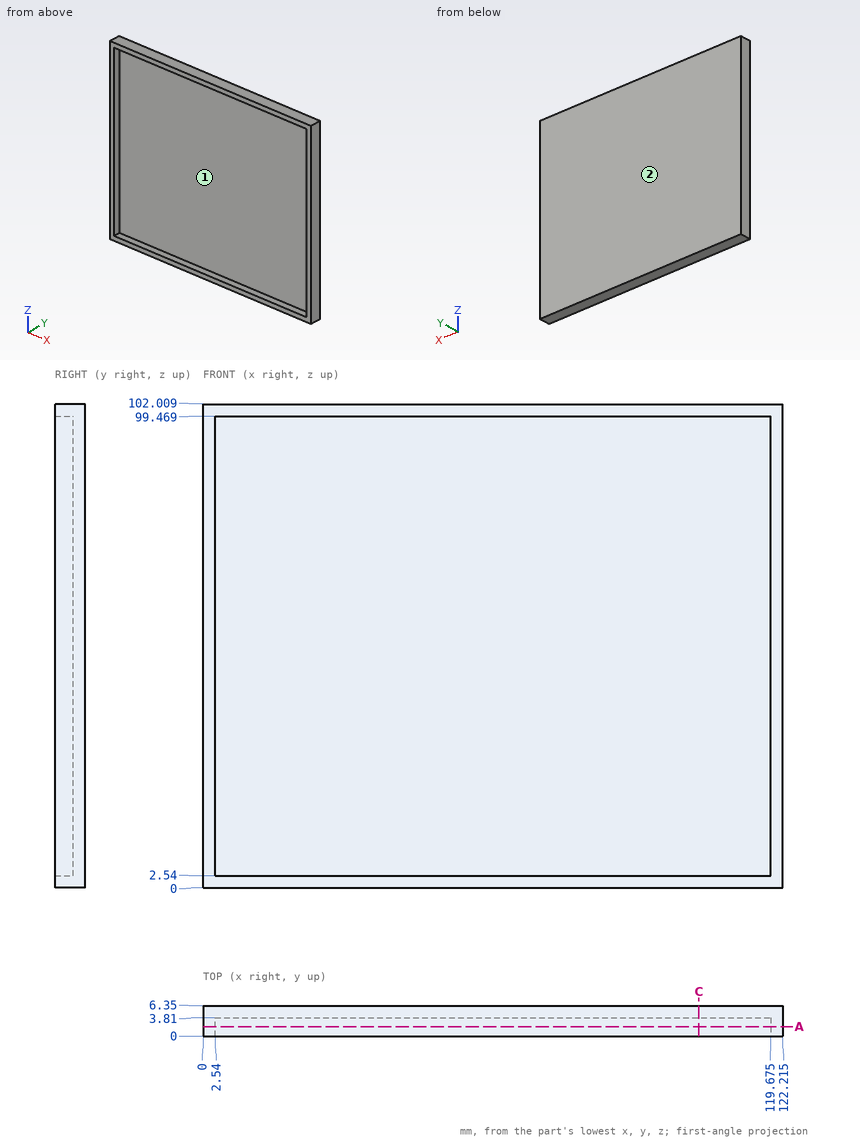
Can you work these out from the drawing? Everything is in mm from the part's minimum corner. Coordinates: 2 decimals unless noted, no trailing zeros. Write each loop counter-clockwise with the first axis right and the second up, starting at its lowest first coordinate (ties: lowest second). Pieces come first, ordered by that corner, then holes. Notation, with made-up numbers: (31, 52) -> (88, 52) arc R34 cw to (88, 86) -> close; hole circle Ø3 at (80.5, 22). An arc over 180 degrees is marked (long way). Write each question's results on one line, items separated by ' | '. Start each with the question number.
Item 1: If we section it at C-C, the plane x = 104.5: Write out the boundary of the cut face in (y, z).
Item 2: Thinking about a two-plate mould opening in X: for the marked faces 1 and 2, which applies, released by +X, released by -X, zero draft, split by the parting line, or undercut?
Item 3: Please list where these lines run through material, in increasing order: probe 1 along Z at (x, y) = (92, 0.75); probe 2 along X at (y, z) = (0.5, 10.5) (1 decimal); probe 3 along Y at (x, z) = (29.5, 11).
Item 4: If we section it at A-A, the plane y = 2: Write out the boundary of the cut face in (x, z) (1 decimal), and give its area (3 significant figures).
Item 5: I'm going to push flat-ended pins straight in: P1, Ø1.5, axis at x = 86.5, y = 5.5, coming from the -Z side; P2, Ø12, axis at x = 104.5, z = 11, coming from the -Y side. Where does each tip first touch, or does it pass through?
Answer block:
1) outline: (0, 0) -> (6.35, 0) -> (6.35, 102.01) -> (0, 102.01) -> (0, 99.47) -> (3.81, 99.47) -> (3.81, 2.54) -> (0, 2.54) -> close
2) face 1: undercut | face 2: zero draft
3) probe 1: 0 to 2.54, 99.47 to 102.01 | probe 2: 0 to 2.5, 119.7 to 122.2 | probe 3: 3.81 to 6.35
4) outline: (0, 0) -> (122.2, 0) -> (122.2, 102) -> (0, 102) -> close; hole (2.5, 2.5) -> (119.7, 2.5) -> (119.7, 99.5) -> (2.5, 99.5) -> close | area: 1,110 mm²
5) P1: z = 0 | P2: y = 3.81
